Build history of the part. All positions in model axes, mm. Round coordinates to 2 decimals unless told otherwise and drop trailing zeros. Order: outer loops, then holes, each group sorted by start corner. A loop starts at its lowest first (then second) coordinate and runs counter-clockwise, first axis right, second up. Notation, with made-up numbers: (74, 7) -> (131, 7) arc R24 cw to (131, 18) -> close; hole circle Ø7 at (52.25, 9). An arc over 180 degrees is marked (long way). Answer as a JSON object with one key per item and string values.
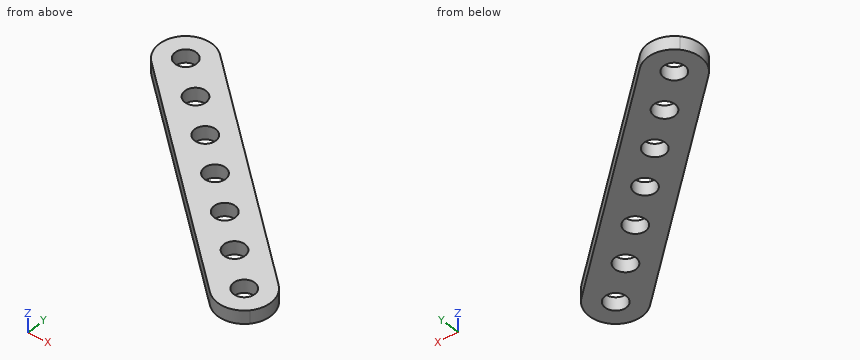
Autodesk Inventor part; units mm, degrees
ref_plane "YZ Plane" through (0, 0, 0) normal (1, 0, 0) x (0, 1, 0)
ref_plane "XZ Plane" through (0, 0, 0) normal (0, 1, 0) x (-1, 0, 0)
ref_plane "XY Plane" through (0, 0, 0) normal (0, 0, 1) x (1, 0, 0)
sketch "Sketch1" plane through (0, 0, 0) normal (0, 0, 1) x (1, 0, 0)
  line L0 (4.2818, -5.6498) -> (9.6498, 0.2818)
  line L1 (9.6498, 0.2818) -> (-27.4231, 33.8318)
  line L2 (-27.4231, 33.8318) -> (-32.7911, 27.9001)
  line L3 (-32.7911, 27.9001) -> (4.2818, -5.6498)
  circle A0 centre (4, 0) radius 1.6
  circle A1 centre (4, 0) radius 1.6
  circle A2 centre (-1.1902, 4.697) radius 1.6
  circle A3 centre (-6.3804, 9.394) radius 1.6
  circle A4 centre (-11.5706, 14.091) radius 1.6
  circle A5 centre (-16.7608, 18.788) radius 1.6
  circle A6 centre (-21.951, 23.485) radius 1.6
  circle A7 centre (-27.1413, 28.182) radius 1.6
  point P0 (0, 0)
  dimension "d0" = 8
  dimension "d1" = 4
  dimension "d2" = 4
  dimension "d5" = 7
  dimension "d10" = 4
extrude "Extrusion1" add sketch "Sketch1" along normal blind 2
fillet "Fillet1" radius 4 4 edges at (-32.7911, 27.9001, 1) (-27.4231, 33.8318, 1) (4.2818, -5.6498, 1) (9.6498, 0.2818, 1)
equation "\"d1\" = 0.5 * d0"
properties part number "control-arm"
1) Cut at B-B, the plane z = 0.5. Count the separate pieces of the cut face and the enclosed holes in it, plus the area to 3 significant figures.
Checked values:
{"separate pieces": "1", "enclosed holes": "7", "area": "330 mm²"}
2) Flat gauge pin, fed straight in: pin 1 Ø1 at (y, z) = (22, 2) entering from -X. Where does the tip first touch, or does it go through?
Checked values:
{"pin 1": "stops at x = -26.82"}
3) Cut at A-A, the plane y = 0. Give the cut face in (x, z), plus the area to 3 significant figures.
Checked values:
{"outline": "(-1.96, 0) -> (2.4, 0) -> (2.4, 2) -> (-1.96, 2) -> close; (5.6, 0) -> (8, 0) -> (8, 2) -> (5.6, 2) -> close", "area": "13.5 mm²"}
4) Cut at C-C, the plane x = 4. Give the cut face in (y, z), plus the area to 3 significant figures.
Checked values:
{"outline": "(-4, 0) -> (-1.6, 0) -> (-1.6, 2) -> (-4, 2) -> close; (1.6, 0) -> (5.39, 0) -> (5.39, 2) -> (1.6, 2) -> close", "area": "12.4 mm²"}
5) Probe L1, parallel to X at y = 18, z = 0.45; L2, parallel to Y at x = -26, z = 0.8; L3, parallel to Y at x = 3, z = 0.8. List the from-to ranges inside material, lowest first. Write a range as from..to.
Checked values:
{"L1": "x = -21.85..-18.15, -15.37..-9.93", "L2": "y = 21.75..27.06, 29.3..32.02", "L3": "y = -3.87..-1.25, 1.25..6.3"}
